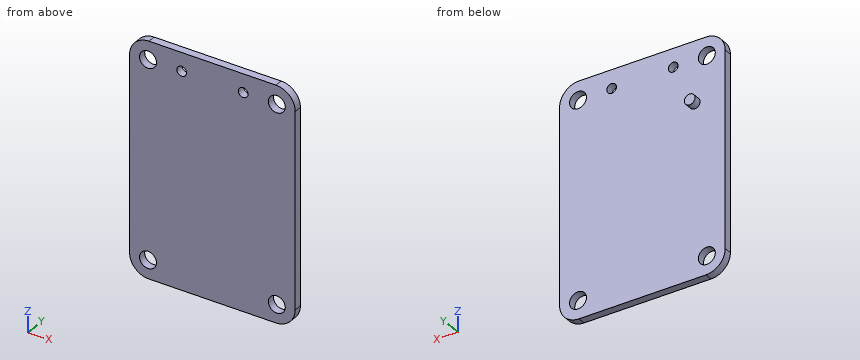
```python
from build123d import *

# Parameters (mm, degrees)
SKETCH1_R           = 1.75
BOSS_EXTRUDE1_DEPTH = 1.62
SKETCH2_R           = 1
CUT_EXTRUDE1_DEPTH  = 1.62
SKETCH3_R           = 1.1
BOSS_EXTRUDE2_DEPTH = 1.6


with BuildPart() as part:
    # Sketch1 → Boss-Extrude1 (new body)
    with BuildSketch(Plane(origin=(0, 0, 0), x_dir=(1, 0, 0), z_dir=(0, 1, 0))):
        with BuildLine():
            Line((30.29, 48.26), (4, 48.26))
            ThreePointArc((4, 48.26), (1.171572875, 47.088427125), (0, 44.26))
            Line((0, 44.26), (0, 4))
            ThreePointArc((0, 4), (1.171572875, 1.171572875), (4, 0))
            Line((4, 0), (30.29, 0))
            ThreePointArc((30.29, 0), (33.118427125, 1.171572875), (34.29, 4))
            Line((34.29, 4), (34.29, 44.26))
            ThreePointArc((34.29, 44.26), (33.118427125, 47.088427125), (30.29, 48.26))
        make_face()
        with Locations((30.48, 44.45)):
            Circle(SKETCH1_R, mode=Mode.SUBTRACT)
        with Locations((3.81, 44.45)):
            Circle(SKETCH1_R, mode=Mode.SUBTRACT)
        with Locations((30.48, 3.81)):
            Circle(SKETCH1_R, mode=Mode.SUBTRACT)
        with Locations((3.81, 3.81)):
            Circle(SKETCH1_R, mode=Mode.SUBTRACT)
    extrude(amount=BOSS_EXTRUDE1_DEPTH)

    # Sketch2 → Cut-Extrude1 (cut)
    with BuildSketch(Plane(origin=(0, 1.62, 0), x_dir=(1, 0, 0), z_dir=(0, 1, 0))):
        with Locations((23.52, 3.81)):
            Circle(SKETCH2_R)
        with Locations((10.77, 3.81)):
            Circle(SKETCH2_R)
    extrude(amount=-CUT_EXTRUDE1_DEPTH, mode=Mode.SUBTRACT)

    # Sketch3 → Boss-Extrude2 (add)
    with BuildSketch(Plane(origin=(0, 1.62, 0), x_dir=(1, 0, 0), z_dir=(0, 1, 0))):
        with Locations((6.3, 12.7)):
            Circle(SKETCH3_R)
    extrude(amount=BOSS_EXTRUDE2_DEPTH)


solid = part.part
```
The listing builds one solid part. Answer for the finished solid, in the listing's coordinates (mm). Coordinates: 2 decimals unless noted, no trailing zeros. Write each loop counter-clockwise with the first axis right and the second up, starting at its lowest first coordinate (ties: lowest second). Pieces come first, ordered by that corner, then holes.
Q1. Find the intervals of material crossed by line 1 along X through (y, z) = (0.5, -3.81); line 2 along Z through (x, y) = (3.81, 1.1); line 3 along X through (y, z) = (1.25, -44.45), in increasing order.
Returned:
line 1: x = 0 to 2.06, 5.56 to 9.77, 11.77 to 22.52, 24.52 to 28.73, 32.23 to 34.29
line 2: z = -48.26 to -46.2, -42.7 to -5.56, -2.06 to 0
line 3: x = 0 to 2.06, 5.56 to 28.73, 32.23 to 34.29
Q2. Section A-A, the plane x = 10.77 is taken. Write down the section's boundary in (y, z).
Returned:
outline: (0, -48.26) - (1.62, -48.26) - (1.62, -4.81) - (0, -4.81) - close; (0, -2.81) - (1.62, -2.81) - (1.62, 0) - (0, 0) - close
Q3. Section C-C, the plane x = 6.3 is taken. Write down the section's boundary in (y, z).
Returned:
outline: (0, -48.26) - (1.62, -48.26) - (1.62, -13.8) - (3.22, -13.8) - (3.22, -11.6) - (1.62, -11.6) - (1.62, 0) - (0, 0) - close
Q4. Given P1, Ø1, axis at x = 14, z = -8, coming from the +Y side, flat-ended and moving along its own axis, determine where the tip first touches the part or whether it passes through.
Returned:
P1: stops at y = 1.62
Q5. Section B-B, the plane z = -12.7 is taken. Write down the section's boundary in (x, y), then the cut area to 3 significant figures.
Returned:
outline: (0, 0) - (34.29, 0) - (34.29, 1.62) - (7.4, 1.62) - (7.4, 3.22) - (5.2, 3.22) - (5.2, 1.62) - (0, 1.62) - close
area: 59.1 mm2
Q6. Section D-D, the plane y = 2.15 is taken. Write down the section's boundary in (x, z).
Returned:
outline: circle Ø2.2 at (6.3, -12.7)
